Read the model definition and answer for the solid it produces. Units are mm, in the model's axes. Round coordinates to 2 decimals unless told otherwise and drop trailing zeros. Order: outer loops, then holes, each group sorted by start corner. A loop starts at its lowest first (then second) coordinate and runs counter-clockwise, first axis right, second up. Notation, with made-up numbers: (-23.5, 8) - (-15.5, 8) arc R15 ccw to (-15.5, 22) - close; hole circle Ø5 at (70.25, 58.25). An arc over 180 degrees is marked (long way). Put each result on its own line as item: value. Start each with the question number.
Q1. Section B-B on x = -5 is taken. Give the vertices of the cut face in (y, z), then the cut area to 3 significant figures.
Q2. Each of these flat-tipped pins is pushed along its axis until it touches: pin 1 Ø0.5 at (y, z) = (1.5, 0.5) entering from -X; pin 2 Ø1 at (x, y) = (9.5, 5) entering from -Z. Where does it stop, or does it pass through?
Q3. Section A-A on y = -6 is taken. Give the vertices of the cut face in (x, z), then the cut area to 3 significant figures.
Q4. Find the intervals of material crossed by line 1 along Z through (x, y) = (-0.25, -10), in increasing order. Write a range as from..to.
from build123d import *

# Parameters (mm, degrees)
BOX015_W     = 2
BOX015_H     = 23
BOX015_DEPTH = 1
BOX014_W     = 2
BOX014_H     = 23
BOX014_DEPTH = 1
BOX013_W     = 2
BOX013_H     = 23
BOX013_DEPTH = 1
BOX012_W     = 2
BOX012_H     = 23
BOX012_DEPTH = 1
BOX016_W     = 2
BOX016_H     = 23
BOX016_DEPTH = 1
BOX011_W     = 23
BOX011_H     = 23
BOX011_DEPTH = 12


with BuildPart() as cube015:
    # Box015 → Box015 (new body)
    with BuildSketch(Plane(origin=(3.5, -11.5, 0), x_dir=(1, 0, 0), z_dir=(0, 0, 1))):
        with Locations((1, 11.5)):
            Rectangle(BOX015_W, BOX015_H)
    extrude(amount=BOX015_DEPTH)


with BuildPart() as cube014:
    # Box014 → Box014 (new body)
    with BuildSketch(Plane(origin=(-1.5, -11.5, 0), x_dir=(1, 0, 0), z_dir=(0, 0, 1))):
        with Locations((1, 11.5)):
            Rectangle(BOX014_W, BOX014_H)
    extrude(amount=BOX014_DEPTH)


with BuildPart() as cube013:
    # Box013 → Box013 (new body)
    with BuildSketch(Plane(origin=(-6.5, -11.5, 0), x_dir=(1, 0, 0), z_dir=(0, 0, 1))):
        with Locations((1, 11.5)):
            Rectangle(BOX013_W, BOX013_H)
    extrude(amount=BOX013_DEPTH)


with BuildPart() as cube012:
    # Box012 → Box012 (new body)
    with BuildSketch(Plane(origin=(-11.5, -11.5, 0), x_dir=(1, 0, 0), z_dir=(0, 0, 1))):
        with Locations((1, 11.5)):
            Rectangle(BOX012_W, BOX012_H)
    extrude(amount=BOX012_DEPTH)


with BuildPart() as fusion011:
    # Box016 → Box016 (new body)
    with BuildSketch(Plane(origin=(8.5, -11.5, 0), x_dir=(1, 0, 0), z_dir=(0, 0, 1))):
        with Locations((1, 11.5)):
            Rectangle(BOX016_W, BOX016_H)
    extrude(amount=BOX016_DEPTH)

    # Fusion011: union Cube015, Cube014, Cube013, Cube012
    add(cube015.part)
    add(cube014.part)
    add(cube013.part)
    add(cube012.part)


with BuildPart() as rubber_pad:
    # Box011 → Box011 (new body)
    with BuildSketch(Plane(origin=(-11.5, -11.5, 0), x_dir=(1, 0, 0), z_dir=(0, 0, 1))):
        with Locations((11.5, 11.5)):
            Rectangle(BOX011_W, BOX011_H)
    extrude(amount=BOX011_DEPTH)

    # Cut002002: cut Fusion011
    add(fusion011.part, mode=Mode.SUBTRACT)


solid = rubber_pad.part
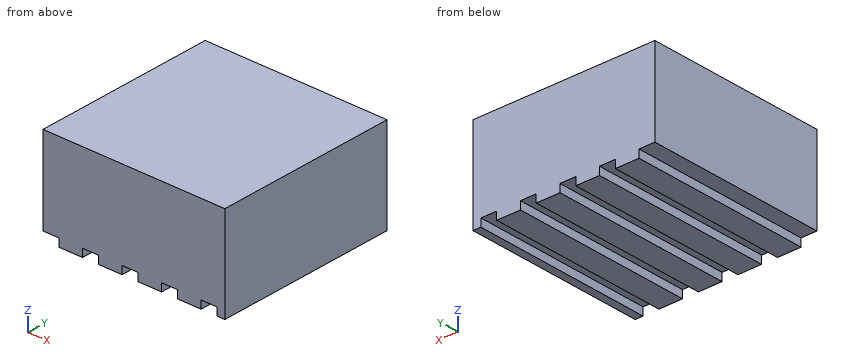
Findings:
1. outline: (-11.5, 1) - (11.5, 1) - (11.5, 12) - (-11.5, 12) - close
1. area: 253 mm2
2. pin 1: x = -9.5
2. pin 2: z = 1
3. outline: (-11.5, 1) - (-9.5, 1) - (-9.5, 0) - (-6.5, 0) - (-6.5, 1) - (-4.5, 1) - (-4.5, 0) - (-1.5, 0) - (-1.5, 1) - (0.5, 1) - (0.5, 0) - (3.5, 0) - (3.5, 1) - (5.5, 1) - (5.5, 0) - (8.5, 0) - (8.5, 1) - (10.5, 1) - (10.5, 0) - (11.5, 0) - (11.5, 12) - (-11.5, 12) - close
3. area: 266 mm2
4. line 1: 1..12
